The model under review builds one solid part; all positions refer to its coordinate system, in mm. Face numbers are marked on the shaded views. Coordinates: 2 decimals unless noted, no trailing zeros. Write each loop counter-clockwise with the first axis right and the second up, starting at its lowest first coordinate (ties: lowest second). Pieces come first, ordered by that corner, then holes. Notation, with made-up numbers: (56, 7) - (63, 7) arc R36 ccw to (63, 42) - close; hole circle Ø3 at (-31, -18.75). An arc over 180 degrees is marked (long way). Put each result on its own line as item: value. Start each with the question number.
Item 1: Consider section D-D on z = 6. Give the boundary of the cut face in (x, y), then the cut area to 3 significant figures.
Item 2: Consider section C-C on z = -32. Give the boundary of the cut face in (x, y).
Item 3: To check wall thickness, follow L1, parallel to X at y = -7.75, z = -24; L2, parallel to Z at x = 0, y = -8.75; L3, parallel to X at y = -7, z = 3. State the ranges of each line that lie inside material, in increasing order. Write a range as [from, to].
Item 4: Consider section B-B on y = -8.25. Give the boundary of the cut face in (x, z), then the cut area to 3 significant figures.
Item 5: Consider section A-A on x = 0. Give the boundary of the cut face in (y, z), then the cut area to 3 significant figures.
Item 6: Mouldability with a two-part tool opening along X and no side actions: class the marked faces 1, 2, 3 and 4 as pulls with the +X half, pulls with the -X half, needs draft (parallel to the pull), parting line crosses it, or undercut.
Item 7: For pin 1 (1 mm diameter, centred on x = -33.5, z = 31, fed in from +Y), flat-tipped, find the tip position at first contact; note if it passes through.
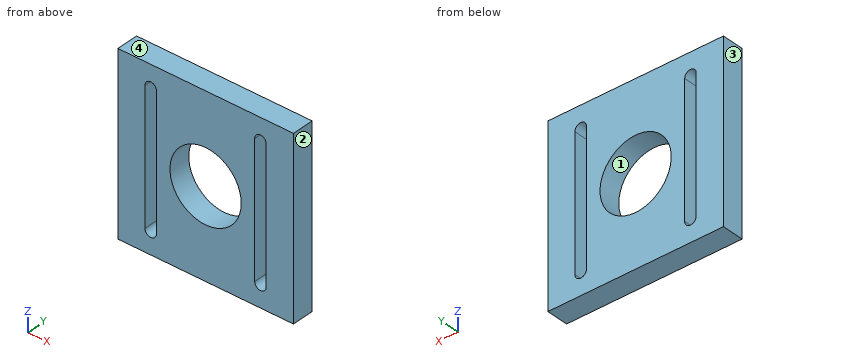
```python
from build123d import *

# Parameters (mm, degrees)
F0_W     = 101.6
F0_H     = 101.6
F0_R     = 20.6121
F1_DEPTH = 12.7
F3_DEPTH = 12.701


with BuildPart() as f1:
    # F0 (on Front) → F1 (new body)
    with BuildSketch(Plane.XZ):
        Rectangle(F0_W, F0_H)
        Circle(F0_R, mode=Mode.SUBTRACT)
    extrude(amount=F1_DEPTH)

    # F2 (on face) → F3 (cut, through all)
    with BuildSketch(Plane.XZ.offset(12.7)):
        with BuildLine():
            Line((35.0901, -38.1), (35.0901, 38.1))
            ThreePointArc((35.0901, 38.1), (31.75, 41.4401), (28.4099, 38.1))
            Line((28.4099, 38.1), (28.4099, -38.1))
            ThreePointArc((28.4099, -38.1), (31.75, -41.4401), (35.0901, -38.1))
        make_face()
        with BuildLine():
            Line((-28.4099, -38.1), (-28.4099, 38.1))
            ThreePointArc((-28.4099, 38.1), (-31.75, 41.4401), (-35.0901, 38.1))
            Line((-35.0901, 38.1), (-35.0901, -38.1))
            ThreePointArc((-35.0901, -38.1), (-31.75, -41.4401), (-28.4099, -38.1))
        make_face()
    extrude(amount=-F3_DEPTH, mode=Mode.SUBTRACT)


solid = f1.part
```
Report:
1. outline: (-50.8, -12.7) - (-35.09, -12.7) - (-35.09, 0) - (-50.8, 0) - close; (-28.41, -12.7) - (-19.72, -12.7) - (-19.72, 0) - (-28.41, 0) - close; (19.72, -12.7) - (28.41, -12.7) - (28.41, 0) - (19.72, 0) - close; (35.09, -12.7) - (50.8, -12.7) - (50.8, 0) - (35.09, 0) - close
1. area: 620 mm²
2. outline: (-50.8, -12.7) - (-35.09, -12.7) - (-35.09, 0) - (-50.8, 0) - close; (-28.41, -12.7) - (28.41, -12.7) - (28.41, 0) - (-28.41, 0) - close; (35.09, -12.7) - (50.8, -12.7) - (50.8, 0) - (35.09, 0) - close
3. L1: [-50.8, -35.09], [-28.41, 28.41], [35.09, 50.8]
3. L2: [-50.8, -20.61], [20.61, 50.8]
3. L3: [-50.8, -35.09], [-28.41, -20.39], [20.39, 28.41], [35.09, 50.8]
4. outline: (-50.8, -50.8) - (50.8, -50.8) - (50.8, 50.8) - (-50.8, 50.8) - close; hole (-35.09, -38.1) arc R3.34 ccw to (-28.41, -38.1) - (-28.41, 38.1) arc R3.34 ccw to (-35.09, 38.1) - close; hole circle Ø41.22 at (0, 0); hole (28.41, -38.1) arc R3.34 ccw to (35.09, -38.1) - (35.09, 38.1) arc R3.34 ccw to (28.41, 38.1) - close
4. area: 7,900 mm²
5. outline: (-12.7, -50.8) - (0, -50.8) - (0, -20.61) - (-12.7, -20.61) - close; (-12.7, 20.61) - (0, 20.61) - (0, 50.8) - (-12.7, 50.8) - close
5. area: 767 mm²
6. face 1: undercut
6. face 2: pulls with the +X half
6. face 3: pulls with the -X half
6. face 4: needs draft
7. pin 1: through
